Verification items for the finished model (mm, model axes). A direction names the side the tool comes from. Give positions to 0.01 mm unless a question says otherwise; leave off trailing zeros. Order: outer loops, then holes, each group sorted by start corner. A loop starts at its lowest first (then second) coordinate and runs counter-clockwise, first axis right, second up. Notation, with made-up numbers: (-25.5, 34) -> (2.5, 34) arc R18 ccw to (2.5, 67) -> close; hole circle Ø9 at (44.5, 8.25). An arc over 180 degrees is marked (long way). Return JSON: item names as keys, results as strings. Group by question number.
(1) Cross-section at A-A on x = 14. Enter the section's corners in (y, z).
(2) Cross-section at C-C on y = -14. Enter the section's corners in (x, z).
(3) Thickness scan on line 1 along Y through (x, z) = (7, -17.25); line 2 along Y through (x, z) = (7.75, -14); line 3 along X through (y, z) = (-5, -13). Record the ranges inside material, lowest first.
(4) Depth check by flat-ended pin: pin 1 Ø1.5 at (x, y) = (9, -9.5) entering from +Z; pin 2 Ø0.5 at (x, y) = (8, 22) entering from +Z (3 decimals); pin 3 Ø8 at (x, z) = (2, -13) entering from +Y; pin 4 Ø5 at (x, y) = (2, 19) entering from -Z. Enter the tip coordinate at first touch or a pass-through.
(5) Tool access check on faces 1 (the face through (8.032, 18.199, -20.925)), 2 (the face through (15.595, 0.301, -16.301)), 3 (the face through (9.44, -15.495, -14.563)), 4 (the face through (15, -0.8, -12)). Record the directions out of +Z, -Z, +X, -X, +Y, -Y that give a thin tool (end or side, any length) a straight path to the whole face; none if there is none.
(6) Cross-section at B-B on z = -11.68. Enter the section's corners in (x, y), then the cut area to 3 significant figures.
from build123d import *

# Parameters (mm, degrees)
SKETCH_2_W      = 15.88
SKETCH_2_H      = 21.21
EXTRUDE_1_DEPTH = 18.5
FILLET_1_R      = 1.37
FILLET_2_R      = 1
SKETCH_3_R      = 4.7625
EXTRUDE_2_DEPTH = 9.53
SKETCH_4_R      = 3.25
EXTRUDE_3_DEPTH = 12.6
CHAMFER_1_SIZE  = 0.5
CHAMFER_2_SIZE  = 1
SKETCH_5_R      = 5.2
EXTRUDE_4_DEPTH = 1.57
SKETCH_6_W      = 1.37
SKETCH_6_H      = 2.36
EXTRUDE_5_DEPTH = 0.8
SKETCH_6_3_W    = 1.37
SKETCH_6_3_H    = 2.36
EXTRUDE_6_DEPTH = 2
SKETCH_7_W      = 0.6
SKETCH_7_H      = 0.6
EXTRUDE_7_DEPTH = 8.636


with BuildPart() as part:
    # Эскиз2 → Бобышка-Вытянуть1 (new body)
    with BuildSketch(Plane(origin=(0, 0, 0), x_dir=(1, 0, 0), z_dir=(0, 1, 0))):
        with Locations((7.94, 10.605)):
            Rectangle(SKETCH_2_W, SKETCH_2_H)
    extrude(amount=EXTRUDE_1_DEPTH)

    # Скругление1
    fillet_1_edges = [part.edges().sort_by_distance(p)[0] for p in [
        (0, 9.25, -21.21),
        (15.88, 9.25, -21.21),
        (15.88, 9.25, 0),
        (0, 9.25, 0),
    ]]
    fillet(fillet_1_edges, radius=FILLET_1_R)

    # Скругление2
    fillet_2_edges = [part.edges().sort_by_distance(p)[0] for p in [
        (0, 0, -10.605),
        (0, 18.5, -10.605),
        (7.94, 0, -21.21),
        (15.88, 0, -10.605),
        (7.94, 0, 0),
        (0.40126371, 0, -0.40126371),
        (15.47873629, 0, -0.40126371),
        (15.47873629, 0, -20.80873629),
        (0.40126371, 0, -20.80873629),
        (7.94, 18.5, -21.21),
        (7.94, 18.5, 0),
        (15.88, 18.5, -10.605),
        (0.40126371, 18.5, -0.40126371),
        (15.47873629, 18.5, -0.40126371),
        (15.47873629, 18.5, -20.80873629),
        (0.40126371, 18.5, -20.80873629),
    ]]
    fillet(fillet_2_edges, radius=FILLET_2_R)

    # Эскиз3 → Бобышка-Вытянуть2 (add)
    with BuildSketch(Plane.XZ):
        with Locations((7.94, -11.68)):
            Circle(SKETCH_3_R)
    extrude(amount=EXTRUDE_2_DEPTH)

    # Эскиз4 → Бобышка-Вытянуть3 (add)
    with BuildSketch(Plane.XZ.offset(9.53)):
        with Locations((7.94, -11.68)):
            Circle(SKETCH_4_R)
    extrude(amount=EXTRUDE_3_DEPTH)

    # Фаска1
    chamfer_1_edges = [part.edges().sort_by_distance(p)[0] for p in [
        (4.69, -22.13, -11.68),
    ]]
    chamfer(chamfer_1_edges, length=CHAMFER_1_SIZE)

    # Фаска2
    chamfer_2_edges = [part.edges().sort_by_distance(p)[0] for p in [
        (3.1775, -9.53, -11.68),
    ]]
    chamfer(chamfer_2_edges, length=CHAMFER_2_SIZE)

    # Эскиз5 → Бобышка-Вытянуть4 (add)
    with BuildSketch(Plane.XZ):
        with Locations((7.94, -11.68)):
            Circle(SKETCH_5_R)
    extrude(amount=EXTRUDE_4_DEPTH)

    # Эскиз6 → Бобышка-Вытянуть5 (add)
    with BuildSketch(Plane.XZ):
        with Locations((15.195, -11.68)):
            Rectangle(SKETCH_6_W, SKETCH_6_H)
    extrude(amount=EXTRUDE_5_DEPTH)

    # Эскиз6<3> → Бобышка-Вытянуть6 (add)
    with BuildSketch(Plane.XZ):
        with Locations((15.195, -11.68)):
            Rectangle(SKETCH_6_3_W, SKETCH_6_3_H)
    extrude(amount=-EXTRUDE_6_DEPTH)

    # Эскиз7 → Бобышка-Вытянуть7 (add)
    with BuildSketch(Plane(origin=(0, 18.5, 0), x_dir=(1, 0, 0), z_dir=(0, 1, 0))):
        with Locations((10.48, 2.455)):
            Rectangle(SKETCH_7_W, SKETCH_7_H)
        with Locations((13.02, 2.455)):
            Rectangle(SKETCH_7_W, SKETCH_7_H)
        with Locations((5.4, 2.455)):
            Rectangle(SKETCH_7_W, SKETCH_7_H)
        with Locations((7.94, 2.455)):
            Rectangle(SKETCH_7_W, SKETCH_7_H)
        with Locations((2.86, 2.455)):
            Rectangle(SKETCH_7_W, SKETCH_7_H)
    extrude(amount=EXTRUDE_7_DEPTH)


solid = part.part
Verdict:
{
 "1": {"outline": "(0, -20.21) arc R1 ccw to (1, -21.21) -> (17.5, -21.21) arc R1 ccw to (18.5, -20.21) -> (18.5, -1) arc R1 ccw to (17.5, 0) -> (1, 0) arc R1 ccw to (0, -1) -> close"},
 "2": {"outline": "circle Ø6.5 at (7.94, -11.68)"},
 "3": {"line 1": "0 to 18.5", "line 2": "-22.13 to 18.5", "line 3": "3.36 to 12.52"},
 "4": {"pin 1": "z = -7.25", "pin 2": "z = -2.155", "pin 3": "y = 18.5", "pin 4": "z = -21.21"},
 "5": {"face 1": "-Z, +X, -X, +Y", "face 2": "-Z, +X, -Y", "face 3": "-Y", "face 4": "+Z, -Z, +X, -Y"},
 "6": {"outline": "(0, 1) arc R1 ccw to (1, 0) -> (2.74, 0) -> (2.74, -1.57) -> (3.18, -1.57) -> (3.18, -8.53) -> (4.18, -9.53) -> (4.69, -9.53) -> (4.69, -21.63) -> (5.19, -22.13) -> (10.69, -22.13) -> (11.19, -21.63) -> (11.19, -9.53) -> (11.7, -9.53) -> (12.7, -8.53) -> (12.7, -1.57) -> (13.14, -1.57) -> (13.14, 0) -> (14.51, 0) -> (14.51, -0.8) -> (15.88, -0.8) -> (15.88, 17.5) arc R1 ccw to (14.88, 18.5) -> (1, 18.5) arc R1 ccw to (0, 17.5) -> close", "area": "467 mm²"}
}
